CAD build for the part. Positions are in the model's coordinates, mm. Face numbers are marked on the shaded views. A direction names the side the tool comes from. Coordinates: 2 decimals unless noted, no trailing zeros. Loops run counter-clockwise (first coordinate to the right, second up) from the corner with the lowest first, then second, coordinate; pieces in that order, holes last. Notation, with made-up numbers: (12.25, 46) -> (59.25, 46) arc R25 cw to (59.25, 59) -> close; hole circle Ø11 at (70, -28). An arc over 180 degrees is marked (long way). Write each question's results on one line, items separated by ' | '.
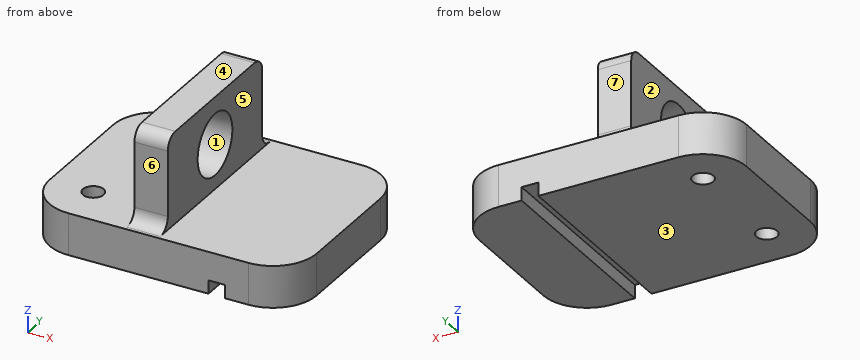
```python
from build123d import *

# Parameters (mm, degrees)
F0_W      = 101.6
F0_H      = 76.2
F1_DEPTH  = 15.875
F2_R      = 3.9624
F3_DEPTH  = 15.875
F4_R      = 16.637
F5_W      = 12.7
F5_H      = 63.5
F6_DEPTH  = 50.8
F7_R      = 5.08
F8_R      = 11.688691
F9_DEPTH  = 25.4
F10_W     = 6.35
F10_H     = 5.08
F11_DEPTH = 101.6


with BuildPart() as f1:
    # F0 (on Top) → F1 (new body)
    with BuildSketch(Plane.XY):
        with Locations((1.375794, 10.99218)):
            Rectangle(F0_W, F0_H)
    extrude(amount=F1_DEPTH)

    # F2 (on face) → F3 (cut)
    with BuildSketch(Plane.XY.offset(15.875)):
        with Locations((-32.787206, 32.45518)):
            Circle(F2_R)
        with Locations((-32.787206, -10.47082)):
            Circle(F2_R)
    extrude(amount=-F3_DEPTH, mode=Mode.SUBTRACT)

    # F4
    f4_edges = [f1.edges().sort_by_distance(p)[0] for p in [
        (-49.424206, 49.09218, 7.9375),
        (52.175794, 49.09218, 7.9375),
        (52.175794, -27.10782, 7.9375),
        (-49.424206, -27.10782, 7.9375),
    ]]
    fillet(f4_edges, radius=F4_R)

    # F5 (on Top) → F6 (join)
    with BuildSketch(Plane.XY):
        with Locations((-4.974206, 10.99218)):
            Rectangle(F5_W, F5_H)
    extrude(amount=F6_DEPTH)

    # F7
    f7_edges = [f1.edges().sort_by_distance(p)[0] for p in [
        (-4.974206, 42.74218, 50.8),
        (-4.974206, -20.75782, 50.8),
        (-4.974206, -20.75782, 15.875),
        (-4.974206, 42.74218, 15.875),
    ]]
    fillet(f7_edges, radius=F7_R)

    # F8 (on face) → F9 (cut)
    with BuildSketch(Plane.YZ.offset(1.375794)):
        with Locations((10.99218, 32.816)):
            Circle(F8_R)
    extrude(amount=-F9_DEPTH, mode=Mode.SUBTRACT)

    # F10 (on face) → F11 (cut)
    with BuildSketch(Plane(origin=(0, 49.09218, 0), x_dir=(-1, 0, 0), z_dir=(0, 1, 0))):
        with Locations((-23.600794, 2.54)):
            Rectangle(F10_W, F10_H)
    extrude(amount=-F11_DEPTH, mode=Mode.SUBTRACT)


solid = f1.part
```
Q1. Cut at D-D on x = -14.5. Write the cut outline in (y, z) (3 decimals).
Results are:
outline: (-27.108, 0) -> (49.092, 0) -> (49.092, 15.875) -> (-27.108, 15.875) -> close
Q2. Cut at B-B on z = 12.5. Write the cut outline in (x, y).
Results are:
outline: (-49.42, -10.47) arc R16.64 ccw to (-32.79, -27.11) -> (35.54, -27.11) arc R16.64 ccw to (52.18, -10.47) -> (52.18, 32.46) arc R16.64 ccw to (35.54, 49.09) -> (-32.79, 49.09) arc R16.64 ccw to (-49.42, 32.46) -> close; hole circle Ø7.92 at (-32.79, -10.47); hole circle Ø7.92 at (-32.79, 32.46)
Q3. Wall check: L1, parallel to X at y = -6.5, z = 35; L2, parallel to Z at x = -16, y = -7 (3 decimals); L3, parallel to Z at x = 21, y = -18 (3 decimals). Give the ranges that are in metal, low to high. Write a range as from..to.
Results are:
L1: -11.32..1.38 | L2: 0..15.875 | L3: 5.08..15.875
Q4. Which spindle directions (+Z, -Z, +X, -X, +Y, -Y) get a long thin tool onto all of the face, cutting with end or side? Do the marked faces 5, 6 and 7. Say none if no direction does.
Results are:
face 5: +Z, +X, +Y, -Y | face 6: +Z, +X, -X, -Y | face 7: +Z, +X, -X, +Y
Q5. Pull direction Z, two halves, no side cores. Call the marked faces 1, 2, 3 and 4: +Z half, -Z half, draft (parallel to the pull), parting line (faces both ways), or undercut.
Results are:
face 1: undercut | face 2: draft | face 3: -Z half | face 4: +Z half
Q6. Cut at C-C on z = 27. Write the cut outline in (x, y).
Results are:
outline: (-11.32, -20.76) -> (1.38, -20.76) -> (1.38, 0.85) -> (-11.32, 0.85) -> close; (-11.32, 21.13) -> (1.38, 21.13) -> (1.38, 42.74) -> (-11.32, 42.74) -> close
Q7. Drop flat-ended pins along their axis: pin 1 (14 mm diameter, centred on x = -3.5, z = 33.5, fed in from -Y); pin 2 (10 mm diameter, centred on x = -5, z = 34, fed in from +Y); pin 3 (9 mm diameter, centred on x = -32.79, y = -10.47, fed in from +Z) (3 decimals). Give the stop position or say it passes through.
Results are:
pin 1: y = -20.76 | pin 2: y = 42.74 | pin 3: z = 15.875
Q8. Cut at A-A on y = 0.5. Write the cut outline in (x, z) (3 decimals).
Results are:
outline: (-49.424, 0) -> (20.426, 0) -> (20.426, 5.08) -> (26.776, 5.08) -> (26.776, 0) -> (52.176, 0) -> (52.176, 15.875) -> (1.376, 15.875) -> (1.376, 27.664) -> (-11.324, 27.664) -> (-11.324, 15.875) -> (-49.424, 15.875) -> close; (-11.324, 37.968) -> (1.376, 37.968) -> (1.376, 50.8) -> (-11.324, 50.8) -> close
